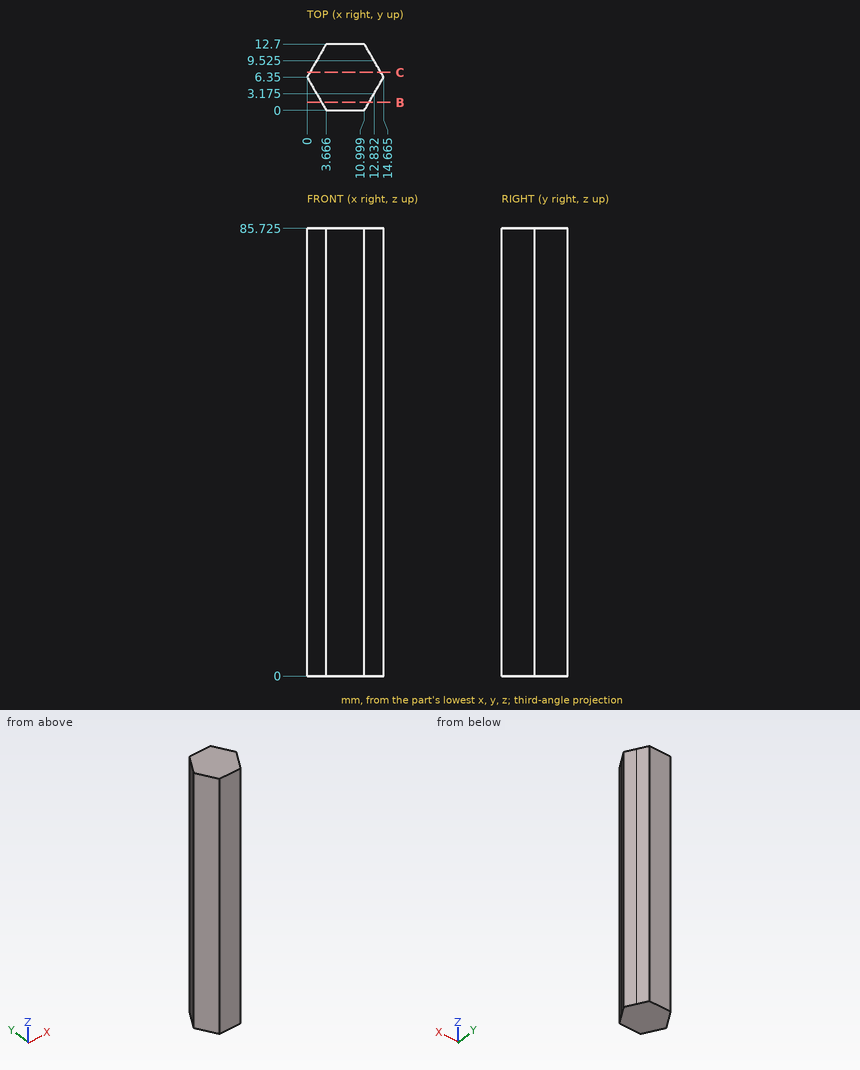
Print and shaded views of the part. All mm, measured from the part's lowest x, y and z. Coordinates: 2 decimals unless noted, no trailing zeros. Order: outer loops, then holes, each group sorted by start corner. A loop starts at its lowest first (then second) coordinate and runs counter-clockwise, first axis right, second up. Notation, with made-up numbers: (19.25, 21.5) - (63.25, 21.5) arc R20 ccw to (63.25, 29.5) - close; hole circle Ø11 at (4, -6). An arc over 180 degrees is marked (long way). Put each result on its own line as item: value.
1. Probe line 1 along Y through (x, z) = (12.75, 81.5) (1 decimal); line 2 along Y through (x, z) = (12.25, 27.5) (1 decimal); line 3 along X through (y, z) = (2.25, 38). List the from-to ranges inside material, lowest first. Write a range as [from, to].
Answer sheet:
line 1: y = [3, 9.7]
line 2: y = [2.2, 10.5]
line 3: x = [2.37, 12.3]
2. Saw through at B-B (y = 1.5). Write the cut outline in (x, z) (1 decimal), and give its area (3 significant figures).
Answer sheet:
outline: (2.8, 0) - (11.9, 0) - (11.9, 85.7) - (2.8, 85.7) - close
area: 777 mm^2
3. Saw through at C-C (y = 7.25). Write the cut outline in (x, z) (1 decimal), and give its area (3 significant figures).
Answer sheet:
outline: (0.5, 0) - (14.1, 0) - (14.1, 85.7) - (0.5, 85.7) - close
area: 1,170 mm^2
4. Drop flat-ended pins along their axis: P1, Ø8, axis at x = 3.5, z = 69, coming from the -Y side; P2, Ø3, axis at y = 1.5, z = 37, coming from the +X side. Give the stop position or say it passes through.
Answer sheet:
P1: stops at y = 0
P2: stops at x = 12.73
